Input: dimensioned drawing with shaded views. Units: mm. Origin: part minimum x, y, z. Coordinates: 2 decimals unless noted, no trailing zeros. One line per question, with ' | ' between items.
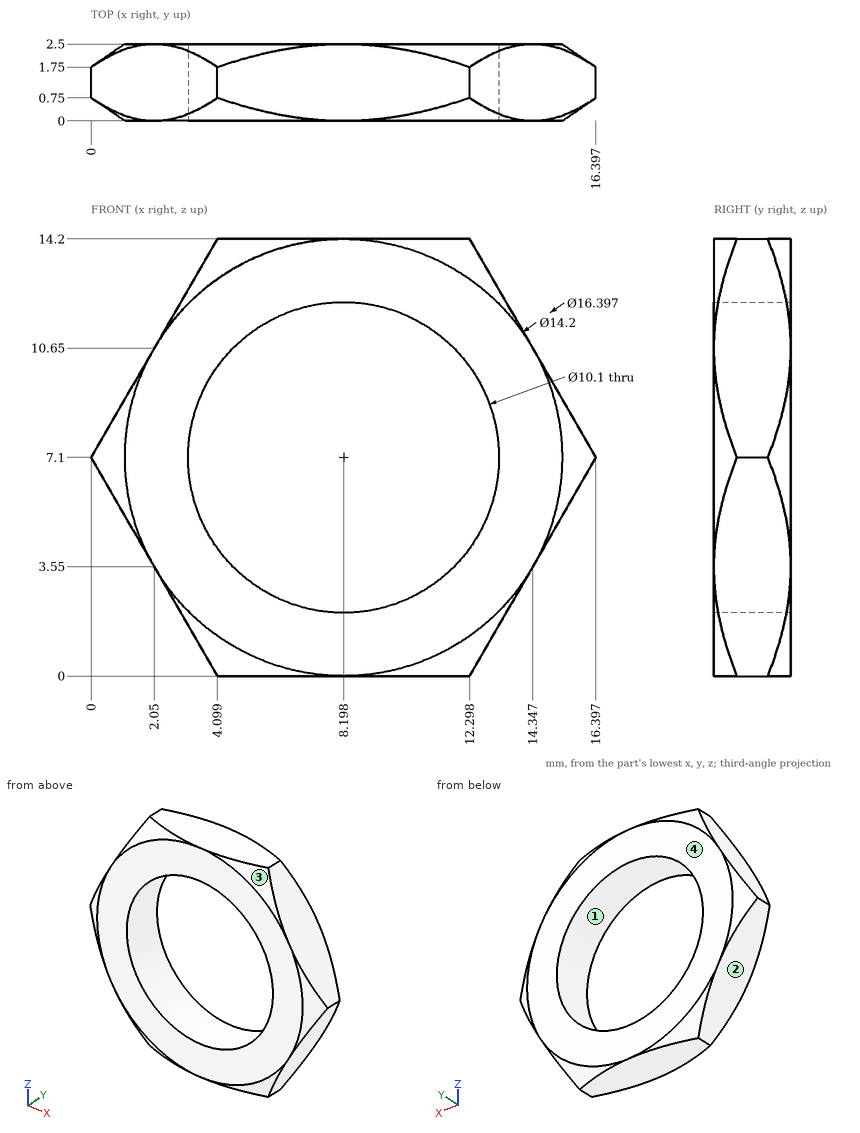
Item 1: Mould query, pull axis Z, two halves, no side actions, for the marked faces 1, 2, 3 and 4. Classes: pulls with the +Z half, pulls with the -Z half, needs draft (parallel to the pull), parting line crosses it, or undercut.
Check sheet entries:
face 1: undercut | face 2: pulls with the -Z half | face 3: pulls with the +Z half | face 4: needs draft
Item 2: Ray query, line 1 along X through (y, z) = (1.15, 3.75) (1 decimal); line 2 along Z through (x, y) = (5.5, 0.45); line 3 along X through (y, z) = (0.3, 10.5) (1 decimal). Return the intervals inside material, ascending. Write a range as [from, to].
Check sheet entries:
line 1: [1.9, 4.4], [12, 14.5] | line 2: [0, 2.83], [11.37, 14.2] | line 3: [2, 4.5], [11.9, 14.4]
Item 3: Pin query (flat end, axial travel): pin 1 Ø1.5 at (x, z) = (6.5, 2.5) entering from -Y; pin 2 Ø1.5 at (y, z) = (0.5, 2.5) entering from +X (1 decimal). Return the tip coordinate at first contact, or that it passes through.
Check sheet entries:
pin 1: y = 0 | pin 2: x = 14.2
